Read the model definition and answer for the solid it produces. Units are mm, in the model's axes. Face numbers are marked on the shaded views. A direction names the side the tool comes from. Give positions to 0.01 mm unless a question says otherwise; leave off trailing zeros. Write each loop counter-clockwise with the first axis right and the second up, starting at its lowest first coordinate (ties: lowest second). Pieces come first, ordered by that corner, then holes. Notation, with made-up numbers: M 66.25,77.5 L 118.25,77.5 A10 ccw 118.25,82.5 Z; hole C 19,-13.75 d6. An arc over 180 degrees is marked long. Use a Markdown table: item, result. Add a question column.
Item 1: For the marked faces 1 and 2, determine the directions among +Z, -Z, +X, -X, +Y, -Y from which every point of the face is accessible in a straight line to the end or side of a thin tool.
Item 2: A cutting plane is placed at C-C on y = 3. Determine the outline of the cut face in (x, z).
Item 3: A cutting plane is placed at B-B on z = 2.25. Determine the outline of the cut face in (x, y) (3 decimals).
Item 4: The mould has two halves that part along X. Classify the marked faces 3, 4 and 5: pulls with the +X half, pulls with the -X half, needs draft (parallel to the pull), parting line crosses it, or undercut.
Item 5: A cutting plane is placed at A-A on y = 1. Determine the outline of the cut face in (x, z).
Item 6: A cutting plane is placed at D-D on x = 4.25. Determine the outline of the cut face in (y, z).
Item 7: Consider probe 1 along X at (y, z) = (4.25, 4.5); probe 2 along X at (y, z) = (2.75, 2.5); probe 3 along Y at (x, z) = (2, 5.75). Determine where each line is inside the solid, lowest interval first. Write a range as [from, to].
Item 8: Given P1, Ø1, axis at x = -1.5, y = 1, coming from the -Z side, flat-ended and moving along its own axis, determine where the tip first touches the part or whether it passes through.
Autodesk Inventor part; units mm, degrees
ref_plane "YZ Plane" through (0, 0, 0) normal (1, 0, 0) x (0, 1, 0)
ref_plane "XZ Plane" through (0, 0, 0) normal (0, 1, 0) x (-1, 0, 0)
ref_plane "XY Plane" through (0, 0, 0) normal (0, 0, 1) x (1, 0, 0)
sketch "Sketch1" plane through (0, 0, 0) normal (0, 0, 1) x (1, 0, 0)
  line L0 (0, 0) -> (4.826, 4.3221)
  line L1 (4.826, 4.3221) -> (10.16, 0)
  line L2 (10.16, 0) -> (11.43, 6.2217)
  line L3 (0, 0) -> (-4.975, 5.229)
  arc A0 (11.43, 6.2217) -> (-4.975, 5.229) centre (5.08, -24.8868) ccw
  circle A1 centre (5.08, -24.8868) radius 25.4 construction
  circle A2 centre (5.08, -24.8868) radius 21.59 construction
  circle A3 centre (5.08, -49.6518) radius 1.5875
  line L4 (5.08, -49.6518) -> (5.08, -46.4768) construction
  line L5 (0, 0) -> (0, -3.2502)
  circle A4 centre (5.08, -24.8868) radius 22.225
  circle A5 centre (5.08, -49.6518) radius 3.81
  dimension "d40" = 43.18
  dimension "d0" = 31.75
  dimension "d2" = 50.8
  dimension "d3" = 29.21
  dimension "d4" = 30
  dimension "d5" = 10.16
  dimension "d6" = 5.334
  dimension "d43" = 3.175
  dimension "d44" = 3.175
  dimension "d53" = 44.45
  dimension "d54" = 7.62
extrude "Extrusion1" add sketch "Sketch1" along normal blind 6.35 contours L3 A0 L2 L1 L0
properties part number "BearingHolder2" material "ABS Plastic"
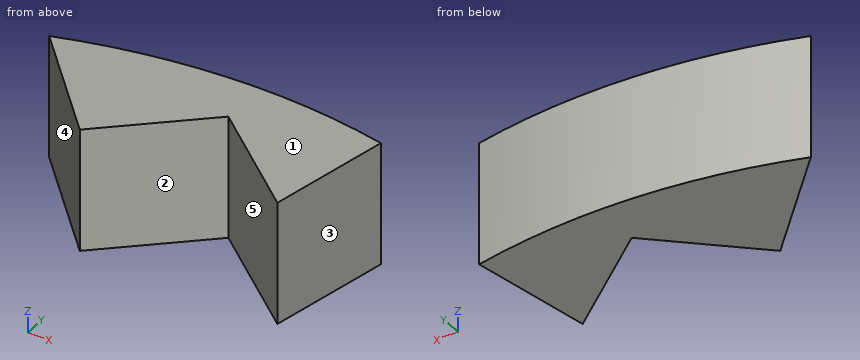
Filled in:
| question | item | result |
|---|---|---|
| 1 | face 1 | +Z, +X, -X, +Y, -Y |
| 1 | face 2 | +Z, -Z, -Y |
| 2 | outline | M -2.85,0 L 3.35,0 L 3.35,6.35 L -2.85,6.35 Z; M 6.46,0 L 10.77,0 L 10.77,6.35 L 6.46,6.35 Z |
| 3 | outline | M -4.975,5.229 L 0,0 L 4.826,4.322 L 10.16,0 L 11.43,6.222 A31.751 ccw Z |
| 4 | face 3 | pulls with the +X half |
| 4 | face 4 | pulls with the -X half |
| 4 | face 5 | undercut |
| 5 | outline | M -0.95,0 L 1.12,0 L 1.12,6.35 L -0.95,6.35 Z; M 8.93,0 L 10.36,0 L 10.36,6.35 L 8.93,6.35 Z |
| 6 | outline | M 3.81,0 L 6.85,0 L 6.85,6.35 L 3.81,6.35 Z |
| 7 | probe 1 | [-4.04, 4.75], [4.91, 11.03] |
| 7 | probe 2 | [-2.62, 3.07], [6.77, 10.72] |
| 7 | probe 3 | [1.79, 6.71] |
| 8 | P1 | z = 0 |
